Part print with two shaded views. Sizes in mm from the minimum x, y, z corner. Round coordinates to 2 decimals unless told otherwise and drop trailing zeros. Write each loop counter-clockwise with the first axis right and the second up, starting at its lowest first coordinate (ties: lowest second). Pieces come first, ordered by that corner, then holes. Notation, with made-up numbers: (77, 0.5) -> (107, 0.5) arc R17 ccw to (107, 14.5) -> close; hole circle Ø8 at (88.25, 79.25). An arc over 180 degrees is marked (long way). Answer as CSV lines item,"result".
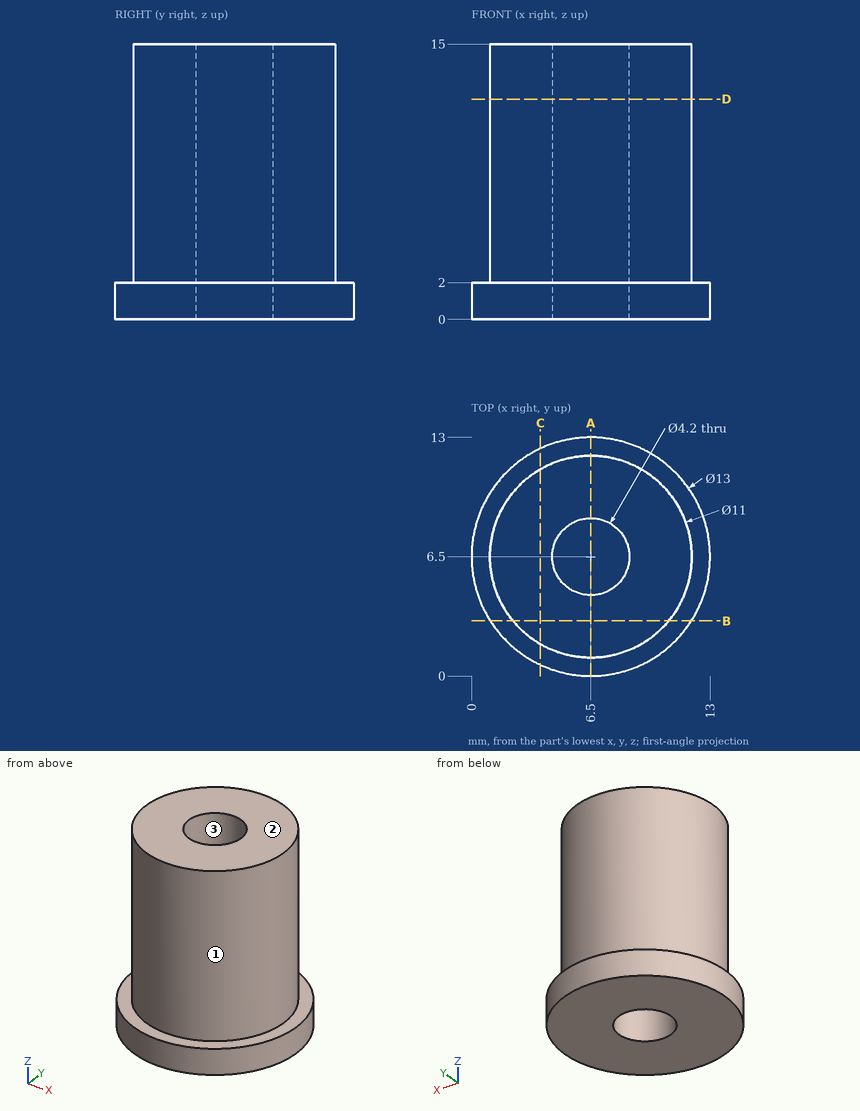
1. Cut at A-A, the plane x = 6.5. Write the cut outline in (y, z), then the cut area to 3 significant figures.
Results found:
outline,"(0, 0) -> (4.4, 0) -> (4.4, 15) -> (1, 15) -> (1, 2) -> (0, 2) -> close; (8.6, 0) -> (13, 0) -> (13, 2) -> (12, 2) -> (12, 15) -> (8.6, 15) -> close"
area,"106 mm2"
2. Cut at D-D, the plane z = 12. Write the cut outline in (x, y).
Results found:
outline,"circle Ø11 at (6.5, 6.5); hole circle Ø4.2 at (6.5, 6.5)"
3. Probe line 1 along X through (y, z) = (6.5, 10.75); line 2 along X through (y, z) = (4.75, 7.25). List the from-to ranges inside material, lowest first.
Results found:
line 1,"x = 1 to 4.4, 8.6 to 12"
line 2,"x = 1.29 to 5.34, 7.66 to 11.71"
4. Cut at C-C, the plane x = 3.75. Write the cut outline in (y, z).
Results found:
outline,"(0.61, 0) -> (12.39, 0) -> (12.39, 2) -> (11.26, 2) -> (11.26, 15) -> (1.74, 15) -> (1.74, 2) -> (0.61, 2) -> close"
5. Cut at B-B, the plane y = 3. Write the cut outline in (x, z).
Results found:
outline,"(1.02, 0) -> (11.98, 0) -> (11.98, 2) -> (10.74, 2) -> (10.74, 15) -> (2.26, 15) -> (2.26, 2) -> (1.02, 2) -> close"
6. Mould opens along Y. For the marked faces 1, 2 and 3 say: +Y half, -Y half, draft (parallel to the pull), parting line (faces both ways), or undercut.
Results found:
face 1,"parting line"
face 2,"draft"
face 3,"undercut"
7. Drop flat-ended pins along their axis: pin 1 Ø4 at (x, y) = (5.5, 5.5) entering from +Z; pin 2 Ø4 at (x, z) = (10.5, 3) entering from +Y; pin 3 Ø1.5 at (y, z) = (6.5, 10.5) entering from +X; pin 4 Ø3 at (x, z) = (9, 10) entering from +Y. Give the stop position or say it passes through.
Results found:
pin 1,"stops at z = 15"
pin 2,"stops at y = 12.59"
pin 3,"stops at x = 12"
pin 4,"stops at y = 11.91"
